from build123d import *

# Parameters (mm, degrees)
SKETCH1_W           = 50
SKETCH1_H           = 30
BOSS_EXTRUDE1_DEPTH = 3
SKETCH2_R           = 2.5
BOSS_EXTRUDE2_DEPTH = 3
SKETCH3_R           = 2.5
CUT_EXTRUDE1_DEPTH  = 3


with BuildPart() as part:
    # Sketch1 → Boss-Extrude1 (new body)
    with BuildSketch(Plane(origin=(0, 0, 0), x_dir=(1, 0, 0), z_dir=(0, 1, 0))):
        Rectangle(SKETCH1_W, SKETCH1_H)
    extrude(amount=BOSS_EXTRUDE1_DEPTH)

    # Sketch2 → Boss-Extrude2 (add)
    with BuildSketch(Plane(origin=(25, 0, 0), x_dir=(0, 0, -1), z_dir=(1, 0, 0))):
        with BuildLine():
            Line((-15, 3), (-15, 43))
            ThreePointArc((-15, 43), (0, 58), (15, 43))
            Line((15, 43), (15, 3))
            Line((15, 3), (-15, 3))
        make_face()
        with Locations((0, 43)):
            Circle(SKETCH2_R, mode=Mode.SUBTRACT)
    boss_extrude2 = extrude(amount=-BOSS_EXTRUDE2_DEPTH)

    # Mirror1: Boss-Extrude2 across plane
    add(boss_extrude2.mirror(Plane(origin=(0, 0, 0), x_dir=(0, 0, 1), z_dir=(1, 0, 0))))

    # Sketch3 → Cut-Extrude1 (cut)
    with BuildSketch(Plane(origin=(0, 3, 0), x_dir=(1, 0, 0), z_dir=(0, 1, 0))):
        with Locations(Location((0, 0, 0), (0, 0, 270))):
            Circle(SKETCH3_R)
    extrude(amount=-CUT_EXTRUDE1_DEPTH, mode=Mode.SUBTRACT)


solid = part.part
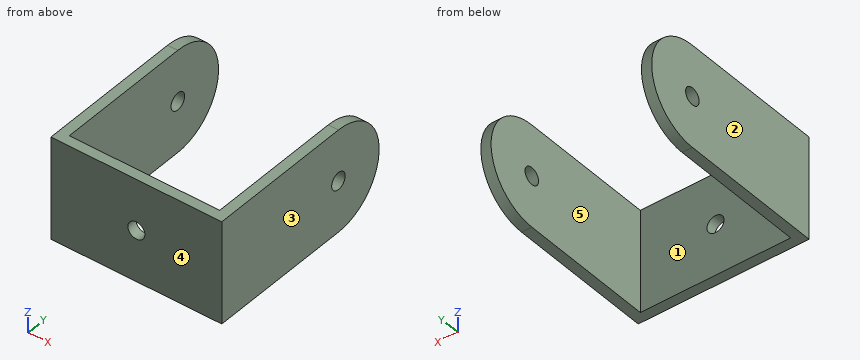
Could you check a few things on this model? Use its own coordinates, in mm. Face numbers are marked on the shaded views. A direction names the side the tool comes from. Give positions to 0.01 mm unless a question says otherwise; leave off trailing zeros. Order: outer loops, then holes, each group sorted by start corner. A loop starts at its lowest first (then second) coordinate and runs counter-clockwise, first axis right, second up. Notation, with made-up numbers: (-36.75, 34.25) - (9.25, 34.25) arc R23 cw to (9.25, 49.25) - close; hole circle Ø10 at (72.5, 8.25). An arc over 180 degrees is marked (long way). One line per item, written item: value. Start each with the question number.
1. Thinking about a two-plate mould opening in X: for the marked faces 3, 4 and 5, which applies, +X half, -X half, draft (parallel to the pull), parting line (faces both ways), or undercut?
2. Imagine slicing it at D-D on z = 3.75. List the corners of the cut face in (x, y) for me.
3. Imagine slicing it at A-A on z = 0. List the corners of the cut face in (x, y) for me.
4. If I drill on probe 1 along Y at (x, z) = (24.1, 0); probe 2 along X at (y, z) = (25, -2.25); probe 3 along X at (y, z) = (1.55, 0), over which ranges is the centre line in solid material (lowest first)?
5. For P1, Ø12, axis at x = 8, z = 1.5, coming from the +Y side, with a flat end and sliding along its axis, tell me the tip position at first contact or that it passes through.
6. Imagine slicing it at B-B on x = 0. List the corners of the cut face in (y, z) for me, plus the area to 3 significant figures.
7. Imagine slicing it at C-C on y = 21. List the corners of the cut face in (x, z) for me, plus the area to 3 significant figures.
8. For the marked faces 1 and 2, which set-ups out of +Z, -Z, +X, -X, +Y, -Y let a thin tool reach every point of the face, with its end or its side?
Values:
1. face 3: +X half
1. face 4: draft
1. face 5: undercut
2. outline: (-25, 0) - (25, 0) - (25, 57.52) - (22, 57.52) - (22, 3) - (-22, 3) - (-22, 57.52) - (-25, 57.52) - close
3. outline: (-25, 0) - (-2.5, 0) - (-2.5, 3) - (-22, 3) - (-22, 40.5) - (-25, 40.5) - close; (-25, 45.5) - (-22, 45.5) - (-22, 58) - (-25, 58) - close; (2.5, 0) - (25, 0) - (25, 40.5) - (22, 40.5) - (22, 3) - (2.5, 3) - close; (22, 45.5) - (25, 45.5) - (25, 58) - (22, 58) - close
4. probe 1: 0 to 40.5, 45.5 to 58
4. probe 2: -25 to -22, 22 to 25
4. probe 3: -25 to -2.5, 2.5 to 25
5. P1: y = 3
6. outline: (0, -15) - (3, -15) - (3, -2.5) - (0, -2.5) - close; (0, 2.5) - (3, 2.5) - (3, 15) - (0, 15) - close
6. area: 75.0 mm²
7. outline: (-25, -15) - (-22, -15) - (-22, 15) - (-25, 15) - close; (22, -15) - (25, -15) - (25, 15) - (22, 15) - close
7. area: 180 mm²
8. face 1: +Z, -Z, +Y
8. face 2: +Z, -Z, -X, +Y, -Y
